```python
from build123d import *

# Parameters (mm, degrees)
TUBE_CLAMP_BASE_EXTRUDE_DEPTH           = 67
TUBE_CLAMP_MOUNTING_PLATE_EXTRUDE_DEPTH = 79
INNER_START                             = -64
INNER_SHELL_DEPTH                       = 64
F_5_0MM_DOWEL_HOLE1_D                   = 5


# Read off the part's stored shape, not the designer's step: Inner Shell
with BuildPart() as part:
    # Tube Clamp Profile → Tube Clamp Base Extrude (new body)
    with BuildSketch(Plane(origin=(0, 0, 0), x_dir=(0, 0, -1), z_dir=(1, 0, 0))):
        with BuildLine():
            Line((-28, 15), (-28, 0))
            ThreePointArc((-28, 0), (0, -28), (28, 0))
            Line((28, 0), (28, 15))
            Line((28, 15), (-28, 15))
        make_face()
    extrude(amount=-TUBE_CLAMP_BASE_EXTRUDE_DEPTH)

    # Sketch1<3> → Tube Clamp Mounting Plate Extrude (add)
    with BuildSketch(Plane(origin=(0, 0, 0), x_dir=(0, 0, -1), z_dir=(1, 0, 0))):
        Polygon((40, 15), (40, 18), (-40, 18), (-40, 15), (-28, 15), (28, 15), align=None)
    extrude(amount=-TUBE_CLAMP_MOUNTING_PLATE_EXTRUDE_DEPTH)

    # Inner Shell outline → Inner Shell (cut)
    with BuildSketch(Plane.YZ.offset(INNER_START)):
        with BuildLine():
            Line((18, -25), (18, 25))
            Line((18, 25), (0, 25))
            ThreePointArc((0, 25), (-25, 0), (0, -25))
            Line((0, -25), (18, -25))
        make_face()
    extrude(amount=INNER_SHELL_DEPTH, mode=Mode.SUBTRACT)

    # Ø5.0mm Dowel Hole1 (through all)
    with Locations(Plane.XZ):
        with Locations((-7.5, -32.5), (-71.5, 32.5), (-7.5, 32.5), (-71.5, -32.5)):
            Hole(F_5_0MM_DOWEL_HOLE1_D / 2)


solid = part.part
```
Source: CAD feature listing. Evaluate the final solid. Frame: model axes, mm. A direction names the side the tool comes from. Round coordinates to 2 decimals unless told otherwise and drop trailing zeros. Loops run counter-clockwise (first coordinate to the right, second up) from the corner with the lowest first, then second, coordinate; pieces in that order, holes last. Notation, with made-up numbers: (39, -1) - (59, -1) arc R4 cw to (59, 6) - close; hole circle Ø2 at (13, 59.25). An arc over 180 degrees is marked (long way). Use CSV: the item, a comma, the result in double quotes.
Q1. Pin query (flat end, axial travel): pin 1 Ø4 at (x, y) = (-10, -19) entering from +Z; pin 2 Ø4 at (x, z) = (-35.5, 13) entering from -Y; pin 3 Ø6 at (x, z) = (-36, -1.5) entering from -Y. Return the tip coordinate at first contact, or that it passes through.
Reported:
pin 1,"z = 22.25"
pin 2,"y = -25.75"
pin 3,"y = -28"
Q2. Section query A-A, the plane z = 32.5. Output: boundary loops of the cut face in (x, y), then the cut area to 3 significant figures.
Reported:
outline,"(-79, 15) - (-74, 15) - (-74, 18) - (-79, 18) - close; (-69, 15) - (-10, 15) - (-10, 18) - (-69, 18) - close; (-5, 15) - (0, 15) - (0, 18) - (-5, 18) - close"
area,"207 mm^2"
Q3. Reachability of faces 1 (the flat face through (-67, -1, 0)), 2 (the flat face through (-32, 9, 25)), 3 (the flat face through (-33, 8, 28)), 4 (the flat face through (-33, 7, -28)) from +Z, -Z, +X, -X, +Y, -Y: full face, straight path, thin tool, end or side. Return the list, or none.
Reported:
face 1,"+Z, -Z, -X, -Y"
face 2,"+X, +Y"
face 3,"+Z, +X, -X, -Y"
face 4,"-Z, +X, -X, -Y"
Q4. Section query D-D, the plane x = -20. Output: boundary loops of the cut face in (y, z).
Reported:
outline,"(0, -28) - (15, -28) - (15, -40) - (18, -40) - (18, -25) - (0, -25) arc R25 cw to (0, 25) - (18, 25) - (18, 40) - (15, 40) - (15, 28) - (0, 28) arc R28 ccw to start"
Q5. Section query C-C, the plane y = 4. Output: boundary loops of the cut face in (x, z).
Reported:
outline,"(-67, -28) - (0, -28) - (0, -25) - (-64, -25) - (-64, 25) - (0, 25) - (0, 28) - (-67, 28) - close"
Q6. Section query B-B, the plane x = -71.5. Output: boundary loops of the cut face in (y, z), then the cut area to 3 significant figures.
Reported:
outline,"(15, -40) - (18, -40) - (18, -35) - (15, -35) - close; (15, -30) - (18, -30) - (18, 30) - (15, 30) - close; (15, 35) - (18, 35) - (18, 40) - (15, 40) - close"
area,"210 mm^2"
Q7. Mould query, pull axis X, two halves, no side actions, for faces 5 (the cylindrical face through (-8.84, 16.52, 34.61)), 6 (the flat face through (-64, -4, 0)), 7 (the cylindrical face through (-33.031, -27.993, 0.616)). Classes: pulls with the +X half, pulls with the -X half, needs draft (parallel to the pull), parting line crosses it, or undercut.
Reported:
face 5,"undercut"
face 6,"pulls with the +X half"
face 7,"needs draft"
Q8. Ray query, line 1 along Z through (x, y) = (-12, 8.5); line 2 along Z through (x, y) = (-7.5, 17.35); line 3 along X through (y, z) = (16, -32). Return the intervals inside material, ascending.
Reported:
line 1,"-28 to -25, 25 to 28"
line 2,"-40 to -35, -30 to -25, 25 to 30, 35 to 40"
line 3,"-79 to -73.95, -69.05 to -9.95, -5.05 to 0"
